Geometry: see drawing. Coordinates: mm, zero at the bounding-box minimum. A direction names the side the tool comes from. Coordinates: 2 decimals unless noted, no trailing zeros. Order: outer loops, then holes, each group sorted by start corner. A loop starts at its lowest first (then second) coordinate and runs counter-clockwise, first axis right, second up. Notation, with made-up numbers: M -26,-27 L 14,-27 A8 cw 14,-20 Z; hole C -40,-12.5 d5. An arc over 180 degrees is marked long. One line per item, written item: value.
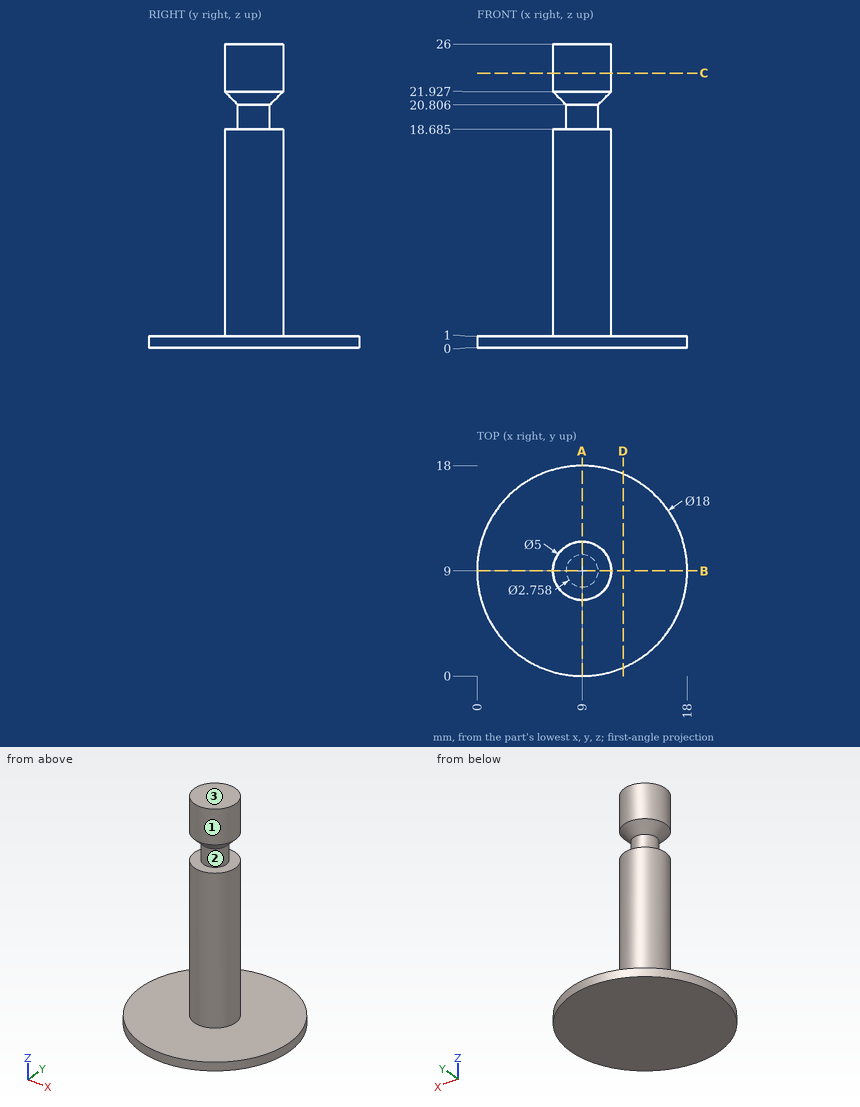
(1) Access query for the marked faces 1, 2 and 3. Directions: +Z, -Z, +X, -X, +Y, -Y. A direction counts if a zero-diameter tool reaches every point of the face in a straight line with its end or side. Return the directions, or none.
Data:
face 1: +Z
face 2: none
face 3: +Z, +X, -X, +Y, -Y
(2) Cut plane A-A on x = 9. Output: boundary loops of the cut face in (y, z) (1 decimal), plus the area to 3 significant figures.
Data:
outline: M 0,0 L 18,0 L 18,1 L 11.5,1 L 11.5,18.7 L 10.4,18.7 L 10.4,20.8 L 11.5,21.9 L 11.5,26 L 6.5,26 L 6.5,21.9 L 7.6,20.8 L 7.6,18.7 L 6.5,18.7 L 6.5,1 L 0,1 Z
area: 137 mm2
(3) Ray query, line 1 (Z direction, x = 13, y = 4.5); line 2 (X direction, y = 9, z = 11.75); line 3 (Z direction, x = 7.75, y = 10) (1 decimal). Return the intervals inside material, ascending. Write a range as from..to.
Data:
line 1: z = 0..1
line 2: x = 6.5..11.5
line 3: z = 0..18.7, 21..26
(4) Cut plane D-D on x = 12.5. Output: boundary loops of the cut face in (y, z).
Data:
outline: M 0.71,0 L 17.29,0 L 17.29,1 L 0.71,1 Z
(5) First-contact query: pin 1 (5 mm diameter, centred on x = 2.5, y = 11, fed in from -Z); pin 2 (5 mm diameter, centred on x = 13, z = 21.5, fed in from +Y); pin 3 (1 mm diameter, centred on x = 7, z = 17.5, fed in from -Y); pin 4 (2 mm diameter, centred on x = 10, y = 2, fed in from +Z). Flat tips, straight axial feed; report the tip coordinate or a pass-through.
Data:
pin 1: stops at z = 0
pin 2: stops at y = 10.97
pin 3: stops at y = 7
pin 4: stops at z = 1
(6) Cut plane C-C on z = 23.5. Output: boundary loops of the cut face in (x, y).
Data:
outline: C 9,9 d5
